Geometry: final body of the model. Coordinates: model frame, mm. A direction names the side the tool comes from. Round coordinates to 2 decimals unless told otherwise and drop trailing zeros. Loops run counter-clockwise (first coordinate to the right, second up) from the corner with the lowest first, then second, coordinate; pieces in that order, holes last. Notation, with made-up numbers: M -18,24.5 L 22,24.5 A8 ccw 22,38.5 Z; hole C 80,7.5 d5. An arc over 180 degrees is marked long. Return JSON: item names as keys, results as strings.
from build123d import *

# Parameters (mm, degrees)
F0_W         = 88.9
F0_H         = 63.5
F1_DEPTH     = 3.174
F2_W         = 88.9
F2_H         = 149.226
F3_DEPTH     = 6.35
F4_W         = 34.926
F4_H         = 33.8644637015
F5_DEPTH     = 6.35
F6_W         = 37.0404637015
F6_H         = 33.8644637015
F7_DEPTH     = 6.35
F8_T4_DEPTH  = 6.35
F9_T4_DEPTH  = 6.35
F10_R        = 8
F11_DEPTH    = 152.401
F10_R_2      = 5
F12_DEPTH    = 25.4
F13_R        = 3.175
F14_DEPTH    = 25.4
F15_DEPTH    = 7
F16_DEPTH    = 7
F17_DEPTH    = 7
F18_DEPTH    = 7
F19_W        = 7.62
F19_H        = 7.62
F20_DEPTH    = 63.5
F21_W        = 7.62
F21_H        = 63.5
F22_DEPTH    = 7.62
F24_T1_DEPTH = 82.55
F25_T1_DEPTH = 82.55
F26_R        = 3.81
F28_R        = 3.175
F29_DEPTH    = 25.4
F30_R        = 8.128
F31_DEPTH    = 25.4
F32_R        = 5.08
F33_DEPTH    = 25.4


# Not quite as in the source:
# - a fillet or chamfer that OpenCascade refuses, or shapes differently, is made with other operations: its cross-section is extruded or revolved along the edge and cut away or added
# - two fillets or chamfers of one size are made in one step


with BuildPart() as f1:
    # F0 (on Front) → F1 (new body)
    with BuildSketch(Plane.XZ):
        with Locations((8.606e-07, -8.4644637015)):
            Rectangle(F0_W, F0_H)
    extrude(amount=-F1_DEPTH)

    # F2 (on face) → F3 (join)
    with BuildSketch(Plane(origin=(0, 0, -40.2144637015), x_dir=(1, 0, 0), z_dir=(0, 0, -1))):
        with Locations((8.606e-07, -77.787)):
            Rectangle(F2_W, F2_H)
    extrude(amount=-F3_DEPTH)

    # F4 (on face) → F5 (join)
    with BuildSketch(Plane.YZ.offset(44.4500008606)):
        with Locations((20.637, -16.9322318508)):
            Rectangle(F4_W, F4_H)
    extrude(amount=-F5_DEPTH)

    # F6 (on face) → F7 (join)
    with BuildSketch(Plane(origin=(-44.4499991394, 0, 0), x_dir=(0, -1, 0), z_dir=(-1, 0, 0))):
        with Locations((-21.6942318508, -16.9322318508)):
            Rectangle(F6_W, F6_H)
    extrude(amount=-F7_DEPTH)

    # F8: chamfer of 38.1 on 1 edges, made by hand


with BuildPart() as f8_tool2:
    # F8_s3 → F8_t4 (new body)
    with BuildSketch(Plane.YZ.offset(-44.4499991394)):
        with BuildLine():
            Line((1.036832967, 1.0776307345), (41.292094436, -39.1776307345))
            Line((41.292094436, -39.1776307345), (42.054094436, -39.1776307345))
            ThreePointArc((42.054094436, -39.1776307345), (40.9764637015, -19.5888153673), (40.9764637015, 0))
            Line((40.9764637015, 0), (40.2144637015, 0.762))
            ThreePointArc((40.2144637015, 0.762), (20.6256483342, 0.762), (1.036832967, 1.8396307345))
            Line((1.036832967, 1.8396307345), (1.036832967, 1.0776307345))
        make_face()
    extrude(amount=F8_T4_DEPTH)

    split(bisect_by=Plane.XZ.offset(-3.174), keep=Keep.BOTTOM)

    split(bisect_by=Plane.XY.offset(-33.8644637015), keep=Keep.TOP)


with BuildPart() as f1_1:
    add(f1.part)

    # F8_t1: cut F8_tool2
    add(f8_tool2.part, mode=Mode.SUBTRACT)

    # F9: chamfer of 38.1 on 1 edges, made by hand


with BuildPart() as f9_tool2:
    # F9_s3 → F9_t4 (new body)
    with BuildSketch(Plane.YZ.offset(44.4500008606)):
        with BuildLine():
            Line((-1.0776307345, 1.0776307345), (39.1776307345, -39.1776307345))
            Line((39.1776307345, -39.1776307345), (39.9396307345, -39.1776307345))
            ThreePointArc((39.9396307345, -39.1776307345), (38.862, -19.5888153673), (38.862, 0))
            Line((38.862, 0), (38.1, 0.762))
            ThreePointArc((38.1, 0.762), (18.5111846327, 0.762), (-1.0776307345, 1.8396307345))
            Line((-1.0776307345, 1.8396307345), (-1.0776307345, 1.0776307345))
        make_face()
    extrude(amount=-F9_T4_DEPTH)

    split(bisect_by=Plane.XZ.offset(-3.174), keep=Keep.BOTTOM)

    split(bisect_by=Plane.XY.offset(-33.8644637015), keep=Keep.TOP)


with BuildPart() as f1_2:
    add(f1_1.part)

    # F9_t1: cut F9_tool2
    add(f9_tool2.part, mode=Mode.SUBTRACT)

    # F10 (on face) → F11 (cut, through all)
    with BuildSketch(Plane.XZ):
        with Locations((-23.4761538258, 0)):
            Circle(F10_R)
    extrude(amount=-F11_DEPTH, mode=Mode.SUBTRACT)

    # F10 (on face) → F12 (cut)
    with BuildSketch(Plane.XZ):
        with Locations((-23.4761538258, 0)):
            Circle(F10_R)
        with Locations((23.2181741801, 0)):
            Circle(F10_R_2)
    extrude(amount=-F12_DEPTH, mode=Mode.SUBTRACT)

    # F13 (on face) → F14 (cut)
    with BuildSketch(Plane.XY.offset(-33.8644637015)):
        with Locations((0, 18.4923222025)):
            Circle(F13_R)
        with Locations((-22.079911083, 59.5920197666)):
            Circle(F13_R)
        with Locations((21.367656067, 59.5920197666)):
            Circle(F13_R)
    extrude(amount=-F14_DEPTH, mode=Mode.SUBTRACT)

    # F15 (add): a face of the model
    f15_faces = [f1_2.faces().sort_by_distance(p)[0] for p in [
        (44.4500008606, 76.2, -38.5634637015),
    ]]
    extrude(f15_faces, amount=F15_DEPTH)

    # F16 (add): a face of the model
    f16_faces = [f1_2.faces().sort_by_distance(p)[0] for p in [
        (-44.4499991394, 1.651, -8.4644637015),
    ]]
    extrude(f16_faces, amount=F16_DEPTH)

    # F17 (cut): a face of the model
    f17_faces = [f1_2.faces().sort_by_distance(p)[0] for p in [
        (38.1000008606, 13.4041545672, -23.6343091343),
    ]]
    extrude(f17_faces, amount=-F17_DEPTH, mode=Mode.SUBTRACT)

    # F18 (cut): a face of the model
    f18_faces = [f1_2.faces().sort_by_distance(p)[0] for p in [
        (-38.0999991394, 14.108975801, -22.9294879005),
    ]]
    extrude(f18_faces, amount=-F18_DEPTH, mode=Mode.SUBTRACT)

    # F19 (on face) → F20 (join)
    with BuildSketch(Plane(origin=(0, 0, -40.2144637015), x_dir=(1, 0, 0), z_dir=(0, 0, -1))):
        with Locations((47.6400008606, -148.59)):
            Rectangle(F19_W, F19_H)
    extrude(amount=-F20_DEPTH)

    # F21 (on face) → F22 (join)
    with BuildSketch(Plane.XZ):
        with Locations((-47.6399991394, -8.4644637015)):
            Rectangle(F21_W, F21_H)
    extrude(amount=-F22_DEPTH)

    # F23: F1 across plane


with BuildPart() as f1_3:
    add(f1_2.part)
    add(f1_2.part.mirror(Plane.YZ))

    # F24: fillet of radius 3.81 on 1 edges, made by hand

    # F24_s2 → F24_t1 (cut)
    with BuildSketch(Plane.XY.offset(-49.7394637015)):
        with BuildLine():
            ThreePointArc((47.6400008606, 0), (50.3340776969, 1.1159231637), (51.4500008606, 3.81))
            Line((51.4500008606, 3.81), (51.4500008606, 0))
            Line((51.4500008606, 0), (47.6400008606, 0))
        make_face()
    extrude(amount=F24_T1_DEPTH, mode=Mode.SUBTRACT)

    # F25: fillet of radius 3.81 on 1 edges, made by hand

    # F25_s2 → F25_t1 (cut)
    with BuildSketch(Plane.XY.offset(-49.7394637015)):
        with BuildLine():
            ThreePointArc((-51.4500008606, 3.81), (-50.3340776969, 1.1159231637), (-47.6400008606, 0))
            Line((-47.6400008606, 0), (-51.4500008606, 0))
            Line((-51.4500008606, 0), (-51.4500008606, 3.81))
        make_face()
    extrude(amount=F25_T1_DEPTH, mode=Mode.SUBTRACT)

    # F26
    f26_edges = [f1_3.edges().sort_by_distance(p)[0] for p in [
        (51.450001, 152.4, -8.464464),
        (-51.450001, 152.4, -8.464464),
    ]]
    fillet(f26_edges, radius=F26_R)

    # F28 (on face) → F29 (cut)
    with BuildSketch(Plane.XY.offset(-33.8644637015)):
        with Locations((28.9712660015, 128.3781081438)):
            Circle(F28_R)
        with Locations((-28.9712660015, 128.3781081438)):
            Circle(F28_R)
    extrude(amount=-F29_DEPTH, mode=Mode.SUBTRACT)

    # F30 (on face) → F31 (cut)
    with BuildSketch(Plane.XZ):
        with Locations((-23.2181741801, 0)):
            Circle(F30_R)
    extrude(amount=-F31_DEPTH, mode=Mode.SUBTRACT)

    # F32 (on face) → F33 (cut)
    with BuildSketch(Plane.XZ):
        with Locations((23.2181741801, 0)):
            Circle(F32_R)
    extrude(amount=-F33_DEPTH, mode=Mode.SUBTRACT)


solid = f1_3.part
Q1. Pull-direction query (X, two-part tool) for faces 6 (the cylindrical face through (50.304, 1.086, -8.909)), 7 (the cylindrical face through (-24.542, 59.527, -36.995)), 8 (the cylindrical face through (28.558, 131.526, -36.995)), 9 (the flat face through (-1, 2, 23.286)); classes: pulls with the +X half, pulls with the -X half, needs draft (parallel to the pull), parting line crosses it, or undercut.
Determined:
{"face 6": "pulls with the +X half", "face 7": "undercut", "face 8": "undercut", "face 9": "needs draft"}
Q2. Section query A-A (x = 0). Output: boundary loops of the cut face in (y, z), plus the area to 3 significant figures.
Determined:
{"outline": "M 0,-40.21 L 15.32,-40.21 L 15.32,-33.86 L 3.17,-33.86 L 3.17,23.29 L 0,23.29 Z; M 21.67,-40.21 L 152.4,-40.21 L 152.4,-33.86 L 21.67,-33.86 Z", "area": "1,110 mm^2"}
Q3. Section query C-C (z = 10.5). Output: boundary loops of the cut face in (x, y).
Determined:
{"outline": "M -51.45,3.81 A3.81 ccw -47.64,0 L 47.64,0 A3.81 ccw 51.45,3.81 L 51.45,7.62 L 43.83,7.62 L 43.83,3.17 L -43.83,3.17 L -43.83,7.62 L -51.45,7.62 Z; M -51.45,144.78 L -43.83,144.78 L -43.83,152.4 L -47.64,152.4 A3.81 ccw -51.45,148.59 Z; M 43.83,144.78 L 51.45,144.78 L 51.45,148.59 A3.81 ccw 47.64,152.4 L 43.83,152.4 Z"}
Q4. Reachability of faces 1 (the flat face through (-48, 149, 23.286)), 2 (the flat face through (-48.231, 21.601, -19.486)), 3 (the flat face through (51.45, 70.5, -34.2)), 4 (the flat face through (-45.1, 16, -26)), 5 (the flat face through (43.83, 149, -6)) from +Z, -Z, +X, -X, +Y, -Y: full face, straight path, thin tool, end or side. Return the list, or none.
Determined:
{"face 1": "+Z, +X, -X, +Y, -Y", "face 2": "+Z, +X, -X", "face 3": "+Z, -Z, +X, +Y, -Y", "face 4": "+Z", "face 5": "+Z, +Y"}
Q5. Material intervals for L1, parallel to Z at x = -25.5, y = 42.5; L2, parallel to Y at x = 39, z = 15.5; L3, parallel to Y at x = -47, z = -28.5, sorted ascending.
Determined:
{"L1": "z = -40.21 to -33.86", "L2": "y = 0 to 3.17", "L3": "y = 0 to 30.61, 144.78 to 152.4"}
Q6. Section query B-B (z = 0). Output: boundary loops of the cut face in (x, y).
Determined:
{"outline": "M -51.45,3.81 A3.81 ccw -47.64,0 L -31.35,0 L -31.35,3.17 L -43.83,3.17 L -43.83,7.62 L -51.45,7.62 Z; M -51.45,144.78 L -43.83,144.78 L -43.83,152.4 L -47.64,152.4 A3.81 ccw -51.45,148.59 Z; M -15.09,0 L 18.14,0 L 18.14,3.17 L -15.09,3.17 Z; M 28.3,0 L 47.64,0 A3.81 ccw 51.45,3.81 L 51.45,7.62 L 43.83,7.62 L 43.83,3.17 L 28.3,3.17 Z; M 43.83,144.78 L 51.45,144.78 L 51.45,148.59 A3.81 ccw 47.64,152.4 L 43.83,152.4 Z"}
Q7. Pin query (flat end, axial travel): pin 1 (8 mm diameter, centred on x = -39, y = 35, fed in from +Z); pin 2 (5 mm diameter, centred on x = -5, z = 16, fed in from +Y). Return the tip coordinate at first contact, or that it passes through.
Determined:
{"pin 1": "stops at z = -33.86", "pin 2": "stops at y = 3.17"}
